Autodesk Inventor part; units mm, degrees
ref_plane "YZ Plane" through (0, 0, 0) normal (1, 0, 0) x (0, 1, 0)
ref_plane "XZ Plane" through (0, 0, 0) normal (0, 1, 0) x (-1, 0, 0)
ref_plane "XY Plane" through (0, 0, 0) normal (0, 0, 1) x (1, 0, 0)
sketch "Pushbutton" plane through (0, 0, 0) normal (0, 0, 1) x (1, 0, 0)
  line L0 (-3, -3) -> (3, -3)
  line L1 (3, -3) -> (3, 3)
  line L2 (3, 3) -> (-3, 3)
  line L3 (-3, 3) -> (-3, -3)
  line L4 (-3, -3) -> (3, 3) construction
  line L5 (3, -3) -> (-3, 3) construction
  circle A0 centre (0, 0) radius 1.5
  dimension "d26" = 6
  dimension "d28" = 6
  dimension "d29" = 3
sketch "Grundriss Platine" plane through (0, 0, 0) normal (0, 0, 1) x (1, 0, 0)
  line L0 (50, -31) -> (-50, -31)
  line L1 (-50, -31) -> (-50, 31)
  line L2 (-50, 31) -> (50, 31)
  line L3 (50, 31) -> (50, -31)
  line L4 (50, -31) -> (-50, 31) construction
  line L5 (-50, -31) -> (50, 31) construction
  line L6 (46, -28.52) -> (-46, -28.52) construction
  line L7 (46, -28.52) -> (-46, 28.52) construction
  line L8 (-46, -28.52) -> (46, 28.52) construction
  circle A0 centre (-46, -27) radius 2
  circle A1 centre (46, -27) radius 2
  circle A2 centre (-46, 27) radius 2
  circle A3 centre (46, 27) radius 2
  line L9 (-50, -20.75) -> (-36.6, -20.75)
  line L10 (-36.6, -20.75) -> (-36.6, -4.75)
  line L11 (-36.6, -4.75) -> (-50, -4.75)
  line L12 (-50, -4.75) -> (-50, -20.75)
  line L13 (-23, 6) -> (-15, 6)
  line L14 (-15, 6) -> (-15, -2)
  line L15 (-15, -2) -> (-23, -2)
  line L16 (-23, -2) -> (-23, 6)
  line L17 (30, 6) -> (22, 6)
  line L18 (22, 6) -> (22, 26)
  line L19 (22, 26) -> (30, 26)
  line L20 (30, 26) -> (30, 6)
  point P0 (0, 0)
  dimension "Platine_Breite" = 100
  dimension "Platine_Hoehe" = 62
  dimension "d4" = 4
  dimension "d5" = 4
  dimension "d6" = 4
  dimension "d7" = 4
  dimension "d8" = 4
  dimension "d9" = 4
  dimension "d10" = 4
  dimension "d11" = 4
  dimension "d12" = 4
  dimension "d13" = 10.25
  dimension "d14" = 13.4
  dimension "d15" = 26.25
  dimension "d16" = 29
  dimension "d17" = 27
  dimension "d18" = 8
  dimension "d19" = 8
  dimension "d20" = 37
  dimension "d21" = 8
  dimension "d22" = 72
  dimension "d23" = 20
extrude "Extrusion1" add sketch "Grundriss Platine" along normal blind 2 contours L0 L1 L9 L10 L11 L2 L3
sketch "Bauteile Oberseite" plane through (0, 0, 2) normal (0, 0, 1) x (1, 0, 0)
  line L0 (-50, -31) -> (50, -31)
  line L1 (50, -31) -> (50, 31)
  line L2 (50, 31) -> (-50, 31)
  line L3 (-50, 31) -> (-50, -4.75)
  line L4 (-23, 6) -> (-15, 6)
  line L5 (-50, 0) -> (50, 0) construction
  line L6 (0, 31) -> (0, -31) construction
  line L7 (-3, -3) -> (3, -3)
  line L8 (3, -3) -> (3, 3)
  line L9 (3, 3) -> (-3, 3)
  line L10 (-3, 3) -> (-3, -3)
  line L11 (-3, -3) -> (3, 3) construction
  line L12 (3, -3) -> (-3, 3) construction
  circle A0 centre (0, 0) radius 1.5
  line L13 (-33, -3) -> (-27, -3)
  line L14 (-27, -3) -> (-27, 3)
  line L15 (-27, 3) -> (-33, 3)
  line L16 (-33, 3) -> (-33, -3)
  line L17 (-33, -3) -> (-27, 3) construction
  line L18 (-27, -3) -> (-33, 3) construction
  circle A1 centre (-30, 0) radius 1.5
  line L19 (27, -3) -> (33, -3)
  line L20 (33, -3) -> (33, 3)
  line L21 (33, 3) -> (27, 3)
  line L22 (27, 3) -> (27, -3)
  line L23 (27, -3) -> (33, 3) construction
  line L24 (33, -3) -> (27, 3) construction
  circle A2 centre (30, 0) radius 1.5
  point P0 (-30, 0)
  point P1 (0, 0)
  point P2 (30, 0)
  dimension "d30" = 30
  dimension "d31" = 30
extrude "Extrusion2" add sketch "Bauteile Oberseite" along normal blind 4
extrude "Extrusion3" add sketch "Bauteile Oberseite" along normal blind 12.5 contours A0 | A1 | A2
sketch "Bauteile Unterseite" plane through (0, 0, 0) normal (0, 0, -1) x (-1, 0, 0)
  line L0 (50, -20.75) -> (36.6, -20.75)
  line L1 (36.6, -20.75) -> (36.6, -4.75)
  line L2 (50, 31) -> (50, -4.75)
  line L3 (50, -31) -> (-50, -31)
  line L4 (50, -20.75) -> (50, -31)
  line L5 (36.6, -20.75) -> (15.2, -20.75)
  line L6 (15.2, -20.75) -> (15.2, -4.87)
  line L7 (15.2, -4.87) -> (36.6, -4.87)
  line L8 (36.6, -4.87) -> (36.6, -20.75)
  line L9 (-39.51, -30) -> (11.29, -30)
  line L10 (11.29, -30) -> (11.29, -10)
  line L11 (11.29, -10) -> (-39.51, -10)
  line L12 (-39.51, -10) -> (-39.51, -30)
  line L13 (-39.51, -30) -> (11.29, -10) construction
  line L14 (11.29, -30) -> (-39.51, -10) construction
  line L15 (27.8, 24.05) -> (-5.8, 24.05)
  line L16 (-5.8, 24.05) -> (-5.8, 8.95)
  line L17 (-5.8, 8.95) -> (27.8, 8.95)
  line L18 (27.8, 8.95) -> (27.8, 24.05)
  line L19 (27.8, 24.05) -> (-5.8, 8.95) construction
  line L20 (-5.8, 24.05) -> (27.8, 8.95) construction
  point P0 (0, 0)
  point P1 (-14.11, -20)
  point P2 (11, 16.5)
  dimension "d37" = 15.88
  dimension "d39" = 21.4
  dimension "d40" = 64.11
  dimension "d41" = 11
  dimension "d42" = 20
  dimension "d43" = 50.8
  dimension "d44" = 39
  dimension "d45" = 47.5
  dimension "d46" = 15.1
  dimension "d47" = 33.6
extrude "Extrusion4" add sketch "Bauteile Unterseite" along normal blind 7.7 contours L18 L17 L16 L15
extrude "Extrusion5" add sketch "Bauteile Unterseite" along normal blind 13.5 contours L5 L6 L7 L1
extrude "Extrusion6" add sketch "Bauteile Unterseite" along normal blind 10 contours L12 L11 L10 L9
equation "\"d24\" = Platine_Dicke"
equation "\"Platine_Dicke\" = 2"
equation "\"epsilon\" = 0.1"
equation "\"Wandstaerke\" = 3"
equation "\"Freimass\" = 3"
properties part number "PCB-Model"
Input: part model. Units: mm. Frame: model coordinates. A direction names the side the tool comes from. Round coordinates to 2 decimals unless told otherwise and drop trailing zeros. Loops run counter-clockwise (first coordinate to the right, second up) from the corner with the lowest first, then second, coordinate; pieces in that order, holes last. Notation, with made-up numbers: (-11.75, 6.25) -> (0.25, 6.25) arc R20 cw to (0.25, 18.25) -> close; hole circle Ø3 at (-16.5, -31). An arc over 180 degrees is marked (long way). Write each question's results on one line, items separated by ' | '.
1. Section C-C (x = 46). Return loops of the section in (y, z), and give its area (3 significant figures).
Geometry results:
outline: (-31, 0) -> (-29, 0) -> (-29, 2) -> (-31, 2) -> close; (-25, 0) -> (25, 0) -> (25, 2) -> (-25, 2) -> close; (29, 0) -> (31, 0) -> (31, 2) -> (29, 2) -> close | area: 108 mm2
2. Section B-B (x = -46). Return loops of the section in (y, z), and give its area (3 significant figures).
Geometry results:
outline: (-31, 0) -> (-29, 0) -> (-29, 2) -> (-31, 2) -> close; (-25, 0) -> (-20.75, 0) -> (-20.75, 2) -> (-25, 2) -> close; (-4.75, 0) -> (25, 0) -> (25, 2) -> (-4.75, 2) -> close; (29, 0) -> (31, 0) -> (31, 2) -> (29, 2) -> close | area: 76.0 mm2
3. Ray query, line 1 (Y direction, x = -46, z = 1.6); line 2 (X direction, y = -13, z = -9.5); line 3 (X direction, y = 11.5, z = -2.5). Return the intervals inside material, ascending. Write a range as from..to.
Geometry results:
line 1: -31..-29, -25..-20.75, -4.75..25, 29..31 | line 2: -36.6..-15.2, -11.29..39.51 | line 3: -27.8..5.8
4. Section D-D (y = 14). Return loops of the section in (x, z).
Geometry results:
outline: (-50, 0) -> (-27.8, 0) -> (-27.8, -7.7) -> (5.8, -7.7) -> (5.8, 0) -> (22, 0) -> (22, 2) -> (-50, 2) -> close; (30, 0) -> (50, 0) -> (50, 2) -> (30, 2) -> close
5. Mould query, pull axis Y, two halves, no side actions, for faces 1 (the face through (14, -20, -10)), 2 (the face through (-30, 3, 4)), 3 (the face through (26, 26, 1)). Classes: +Y half, -Y half, draft (parallel to the pull), parting line (faces both ways), or undercut.
Geometry results:
face 1: draft | face 2: +Y half | face 3: undercut
6. Section A-A (y = -27). Return loops of the section in (x, z).
Geometry results:
outline: (-50, 0) -> (-48, 0) -> (-48, 2) -> (-50, 2) -> close; (-44, 0) -> (-11.29, 0) -> (-11.29, -10) -> (39.51, -10) -> (39.51, 0) -> (44, 0) -> (44, 2) -> (-44, 2) -> close; (48, 0) -> (50, 0) -> (50, 2) -> (48, 2) -> close
7. First-contact query: P1, Ø4.5, axis at y = -11, z = -8, coming from the -X side; P2, Ø5, axis at x = -19.5, y = 3, coming from the -Z side; P3, Ø2, axis at y = 0, z = 3.5, coming from the -X side; P4, Ø8.5, axis at x = -19, z = -5.5, coming from the -Y side. Flat tips, straight axial feed; report the tip coordinate or a pass-through.
Geometry results:
P1: x = -36.6 | P2: through | P3: x = -33 | P4: y = -20.75
8. Set-up query: faces 4 (the face through (14, -10, -5)), 5 (the face through (-26, -4.87, -7)), 6 (the face through (-43, -20.75, 1)), 7 (the face through (-33, 0, 4)), 8 (the face through (-3, 0, 4)). Return all of +Z, -Z, +X, -X, +Y, -Y with unobstructed straight access to the full face (end or side cutting, diameter ignored); none if empty.
Geometry results:
face 4: -Z, +X | face 5: -Z, +X, -X | face 6: +Z, -Z, -X | face 7: +Z, -X, +Y, -Y | face 8: +Z, +Y, -Y
